```python
from build123d import *

# Parameters (mm, degrees)
BASE_FLANGE1_DEPTH = 40
CUT_EXTRUDE1_REACH = 52.14
SKETCH6_R          = 2.55
CUT_EXTRUDE2_REACH = 51.84
SKETCH7_R          = 3
FILLET1_R          = 3


# Sheet-metal steps are written as plain solids
with BuildPart() as part:
    # Sketch1 → Base-Flange1 (new body)
    with BuildSketch(Plane.XY):
        with BuildLine():
            Line((0, 20), (0, 3.7366))
            ThreePointArc((0, 3.7366), (-1.094424801, 1.094424801), (-3.7366, 0))
            Line((-3.7366, 0), (-25, 0))
            Line((-25, 0), (-25, 3))
            Line((-25, 3), (-3.7366, 3))
            ThreePointArc((-3.7366, 3), (-3.215745145, 3.215745145), (-3, 3.7366))
            Line((-3, 3.7366), (-3, 20))
            Line((-3, 20), (0, 20))
        make_face()
    extrude(amount=BASE_FLANGE1_DEPTH)

    # Sketch6 → Cut-Extrude1 (cut, up to next)
    with BuildSketch(Plane(origin=(0, 3, 0), x_dir=(1, 0, 0), z_dir=(0, 1, 0)), mode=Mode.PRIVATE) as cut_extrude1_sk1:
        with Locations(Location((-15, -10, 0), (0, 0, 180))):
            Circle(SKETCH6_R)
    cut_extrude1_tool1 = extrude(cut_extrude1_sk1.sketch, amount=-CUT_EXTRUDE1_REACH, mode=Mode.PRIVATE) & part.part
    # Sketch6 → Cut-Extrude1 (cut, up to next)
    with BuildSketch(Plane(origin=(0, 3, 0), x_dir=(1, 0, 0), z_dir=(0, 1, 0)), mode=Mode.PRIVATE) as cut_extrude1_sk2:
        with Locations(Location((-15, -30, 0), (0, 0, 180))):
            Circle(SKETCH6_R)
    cut_extrude1_tool2 = extrude(cut_extrude1_sk2.sketch, amount=-CUT_EXTRUDE1_REACH, mode=Mode.PRIVATE) & part.part
    add(cut_extrude1_tool1.solids().sort_by_distance((-15, 3, 10))[0], mode=Mode.SUBTRACT)
    add(cut_extrude1_tool2.solids().sort_by_distance((-15, 3, 30))[0], mode=Mode.SUBTRACT)

    # Sketch7 → Cut-Extrude2 (cut, up to next)
    with BuildSketch(Plane.ZY.offset(3), mode=Mode.PRIVATE) as cut_extrude2_sk1:
        with Locations((20, 13.7366)):
            Circle(SKETCH7_R)
    cut_extrude2_tool1 = extrude(cut_extrude2_sk1.sketch, amount=-CUT_EXTRUDE2_REACH, mode=Mode.PRIVATE) & part.part
    add(cut_extrude2_tool1.solids().sort_by_distance((-3, 13.7366, 20))[0], mode=Mode.SUBTRACT)

    # Fillet1
    fillet1_edges = [part.edges().sort_by_distance(p)[0] for p in [
        (-1.5, 20, 40),
        (-1.5, 20, 0),
    ]]
    fillet(fillet1_edges, radius=FILLET1_R)


solid = part.part
```
CAD build for the part. Positions are in the model's coordinates, mm. A direction names the side the tool comes from. Coordinates: 2 decimals unless noted, no trailing zeros. Loops run counter-clockwise (first coordinate to the right, second up) from the corner with the lowest first, then second, coordinate; pieces in that order, holes last. Notation, with made-up numbers: (27, -2) - (65, -2) arc R21 ccw to (65, 34) - close; hole circle Ø1 at (53, 1.25). An arc over 180 degrees is marked (long way). Return JSON: item names as keys, results as strings.
1. Mould opens along Z. For faces 1 (the cylindrical face through (-1.52, 16.71, 19.61)), 2 (the cylindrical face through (-12.976, 1.521, 8.448)), 3 (the cylindrical face through (-1.48, 19.14, 39.1)), 4 (the flat face through (-25, 1, 20)) say: released by +Z, released by -Z, zero draft, split by the parting line, or undercut.
Result:
{"face 1": "undercut", "face 2": "undercut", "face 3": "released by +Z", "face 4": "zero draft"}
2. Band-saw the part on D-D (y = 10.25). Give the cut face in (x, z).
Result:
{"outline": "(-3, 0) - (0, 0) - (0, 40) - (-3, 40) - close"}
3. Band-saw the part on B-B (x = -15). Give the cut face in (y, z), and give its area (3 significant figures).
Result:
{"outline": "(0, 0) - (3, 0) - (3, 7.45) - (0, 7.45) - close; (0, 12.55) - (3, 12.55) - (3, 27.45) - (0, 27.45) - close; (0, 32.55) - (3, 32.55) - (3, 40) - (0, 40) - close", "area": "89.4 mm2"}
4. Probe L1, parallel to Z at x = -15, y = 0.85; L2, parallel to Y at x = -8, z = 29.5; L3, parallel to X at y = 16, z = 12.5. List the from-to ranges inside material, lowest first. Write a range as from..to.
Result:
{"L1": "z = 0..7.45, 12.55..27.45, 32.55..40", "L2": "y = 0..3", "L3": "x = -3..0"}
5. 3-axis set-ups, long thin cutter, end or side, ignore diameter. For faces 5 (the flat face through (-14, 0, 20)), 6 (the flat face through (-15, 3, 20)): which of +Z, -Z, +X, -X, +Y, -Y reach the whole face in a straight line?
Result:
{"face 5": "+Z, -Z, +X, -X, -Y", "face 6": "+Z, -Z, -X, +Y"}
6. Band-saw the part on C-C (y = 15.75). Give the cut face in (x, z).
Result:
{"outline": "(-3, 0) - (0, 0) - (0, 17.78) - (-3, 17.78) - close; (-3, 22.22) - (0, 22.22) - (0, 40) - (-3, 40) - close"}
7. Band-saw the part on A-A (z = 30). Give the cut face in (x, y).
Result:
{"outline": "(-25, 0) - (-17.55, 0) - (-17.55, 3) - (-25, 3) - close; (-12.45, 0) - (-3.74, 0) arc R3.74 ccw to (0, 3.74) - (0, 20) - (-3, 20) - (-3, 3.74) arc R0.74 cw to (-3.74, 3) - (-12.45, 3) - close"}
8. Drop flat-ended pins along their axis: pin 1 (8 mm diameter, centred on x = -15, z = 30, fed in from +Y); pin 2 (8 mm diameter, centred on y = 15.5, z = 35, fed in from -X); pin 3 (12 mm diameter, centred on x = -16.5, y = 10, fed in from +Z). Give the stop position or say it passes through.
Result:
{"pin 1": "stops at y = 3", "pin 2": "stops at x = -3", "pin 3": "passes through"}
